```python
from build123d import *

# Parameters (mm, degrees)
SKETCH_R          = 32.25
PAD_DEPTH         = 2.13
SKETCH004_R       = 1.25
SKETCH004_R_2     = 2
POCKET001_DEPTH   = 5
CHAMFER_SIZE      = 1
SKETCH001_R       = 19.2
PAD001_DEPTH      = 1.5
SKETCH003_W       = 13.85
SKETCH003_H       = 6.2
POCKET_DEPTH      = 2.131
POCKET_DEPTH_BACK = 1.501
SKETCH009_R       = 18
POCKET002_DEPTH   = 2
PAD002_DEPTH      = 21


with BuildPart() as part:
    # Sketch → Pad (new body)
    with BuildSketch(Plane.XY):
        Circle(SKETCH_R)
    extrude(amount=PAD_DEPTH)

    # Sketch004 → Pocket001 (cut)
    with BuildSketch(Plane.XY.offset(2.13)):
        with Locations((0, 27)):
            Circle(SKETCH004_R)
        with Locations((19.445436, 19.445436)):
            Circle(SKETCH004_R_2)
        with Locations((27, 0)):
            Circle(SKETCH004_R)
        with Locations((0, -27)):
            Circle(SKETCH004_R)
        with Locations((-19.445436, -19.445436)):
            Circle(SKETCH004_R_2)
        with Locations((-19.445436, 19.445436)):
            Circle(SKETCH004_R_2)
        with Locations((19.445436, -19.445436)):
            Circle(SKETCH004_R_2)
        with Locations((-26.994671, -0.536434)):
            Circle(SKETCH004_R)
    extrude(amount=-POCKET001_DEPTH, mode=Mode.SUBTRACT)

    # Chamfer
    chamfer_edges = [part.edges().sort_by_distance(p)[0] for p in [
        (25.75, 0, 2.13),
        (-1.25, 27, 2.13),
        (-28.244671, -0.536434, 2.13),
        (-1.25, -27, 2.13),
    ]]
    chamfer(chamfer_edges, length=CHAMFER_SIZE)

    # Sketch001 → Pad001 (join)
    with BuildSketch(Plane.XY.offset(2.13)):
        Circle(SKETCH001_R)
    extrude(amount=PAD001_DEPTH)

    # Sketch003 → Pocket (cut, two sides)
    with BuildSketch(Plane.XY.offset(2.13)) as pocket_sk:
        Rectangle(SKETCH003_W, SKETCH003_H)
        with Locations((0, -10.7)):
            Rectangle(SKETCH003_W, SKETCH003_H)
        with Locations((0, 10.7)):
            Rectangle(SKETCH003_W, SKETCH003_H)
    extrude(amount=-POCKET_DEPTH, mode=Mode.SUBTRACT)
    extrude(pocket_sk.sketch, amount=POCKET_DEPTH_BACK, mode=Mode.SUBTRACT)

    # Sketch009 → Pocket002 (cut)
    with BuildSketch(Plane.XY):
        Circle(SKETCH009_R)
    extrude(amount=-POCKET002_DEPTH, mode=Mode.SUBTRACT)

    # Sketch006 → Pad002 (join)
    with BuildSketch(Plane(origin=(0, 0, 0), x_dir=(0.866025, 0.5, 0), z_dir=(0, 0, 1))):
        with BuildLine():
            ThreePointArc((-1.804633, 22.427512), (-19.485572, 11.25), (-20.325112, -9.650898))
            ThreePointArc((-20.325112, -9.650898), (-20.45119, -11.8075), (-18.520479, -12.776614))
            ThreePointArc((-18.520479, -12.776614), (0, -22.5), (18.520479, -12.776614))
            ThreePointArc((18.520479, -12.776614), (20.45119, -11.8075), (20.325112, -9.650898))
            ThreePointArc((20.325112, -9.650898), (19.485572, 11.25), (1.804633, 22.427512))
            ThreePointArc((1.804633, 22.427512), (0, 23.615), (-1.804633, 22.427512))
        make_face()
        with BuildLine():
            ThreePointArc((-1.860528, 21.017812), (-18.273136, 10.55), (-19.132223, -8.897642))
            ThreePointArc((-17.271696, -12.120171), (-17.04771, -9.8425), (-19.132223, -8.897642))
            ThreePointArc((-17.271696, -12.120171), (-16.59064, -13.036896), (-15.860983, -13.915431))
            Line((-14.58548, -11.706194), (-15.860983, -13.915431))
            Line((-13.892659, -12.106194), (-14.58548, -11.706194))
            Line((-15.29504, -14.53519), (-13.892659, -12.106194))
            ThreePointArc((-15.29504, -14.53519), (1.560407, -21.042223), (17.271696, -12.120171))
            ThreePointArc((19.132223, -8.897642), (17.04771, -9.8425), (17.271696, -12.120171))
            ThreePointArc((19.132223, -8.897642), (19.003303, 9.169759), (4.940323, 20.513488))
            Line((4.940323, 20.513488), (3.537942, 18.084493))
            Line((3.537942, 18.084493), (2.845122, 18.484493))
            Line((2.845122, 18.484493), (4.120625, 20.69373))
            ThreePointArc((4.120625, 20.69373), (2.994963, 20.886364), (1.860528, 21.017812))
            ThreePointArc((-1.860528, 21.017812), (0, 19.685), (1.860528, 21.017812))
        make_face(mode=Mode.SUBTRACT)
    extrude(amount=-PAD002_DEPTH)


solid = part.part
```
Can you work these out from the model? Positions are in its coordinate system, mm. A direction names the side the tool comes from. Round coordinates to 2 decimals unless told otherwise and drop trailing zeros. Loops run counter-clockwise (first coordinate to the right, second up) from the corner with the lowest first, then second, coordinate; pieces in that order, holes last. Notation, with made-up numbers: M 82,-36.75 L 107,-36.75 A33 cw 107,-7.75 Z; hole C 8,33 d11. An arc over 180 degrees is marked long. Answer as a JSON object with one key per item and string values. Group by question number.
Q1. Imagine slicing it at A-A, the plane z = -2.75. Please give me the cut outline in (x, y) (3 decimals).
Q2. Will these pins go through, and if not, where does the flat tip stop? pin 1 (8 mm diameter, centred on y = 16, z = -10, fed in from -X); pin 2 (2 mm diameter, centred on y = -19, z = -14, fed in from -X); pin 3 (4.5 mm diameter, centred on x = -19.45, y = -19.45, fed in from +Z).
Q3. On a 3-axis mill with a long thin cutter (end or side, diameter ignored), from which of +Z, -Z, +X, -X, +Y, -Y can I reach the whole of each face in a straight line? I mean faces 3 (the flat face through (-5.978, 19, -10)), 4 (the cylindrical face through (11.513, 19.332, -10.353)), 5 (the flat face through (6.925, -11, 2)), 6 (the cylindrical face through (10.985, -19.636, -10.353)). Say none if no direction works.
Q4. Please list where these lines run through material, in increasing order: L1, parallel to X at y = -19, z = -5.5; L2, parallel to Z at x = 21.5, y = -13; L3, parallel to Z at x = -9, y = 16.
Q5. Imagine slicing it at C-C, the plane y = -27. Please give me the cut outline in (x, z), then the cut area to 3 significant figures.
Q6. We'd pull the mould along X, two halves only. Please class faces 1 (the flat face through (0, -7.6, 2)), 2 (the flat face through (-6.6, -18.8, -21)): +X half, -X half, draft (parallel to the pull), parting line (faces both ways), or undercut.
Q7. Imagine slicing it at B-B, the plane x = -5. Please give me the cut outline in (y, z).
Findings:
{
 "1": {"outline": "M -12.777,-18.52 A1.965 ccw -9.651,-20.325 A22.5 ccw 22.428,-1.805 A1.965 ccw 22.428,1.805 A22.5 ccw -9.651,20.325 A1.965 ccw -12.777,18.52 A22.5 ccw Z; hole M -12.12,-17.272 A1.965 cw -8.898,-19.132 A21.1 ccw -6.778,-19.982 L -6.778,-17.431 L -5.978,-17.431 L -5.978,-20.235 A21.1 ccw 21.018,-1.861 A1.965 cw 21.018,1.861 A21.1 ccw -5.978,20.235 L -5.978,17.431 L -6.778,17.431 L -6.778,19.982 A21.1 ccw -8.898,19.132 A1.965 cw -12.12,17.272 A21.1 ccw Z"},
 "2": {"pin 1": "stops at x = -19.03", "pin 2": "stops at x = -13.5", "pin 3": "stops at z = 2.13"},
 "3": {"face 3": "-Z", "face 4": "-Z, +Y", "face 5": "+Z, -Z", "face 6": "-Z, -Y"},
 "4": {"L1": "x = -12.77 to -8.88, -6.78 to -5.98, 9.18 to 12.05", "L2": "z = 0 to 2.13", "L3": "z = 0 to 3.63"},
 "5": {"outline": "M -17.64,0 L -1.25,0 L -1.25,1.13 L -2.25,2.13 L -17.64,2.13 Z; M 1.25,0 L 17.64,0 L 17.64,2.13 L 2.25,2.13 L 1.25,1.13 Z", "area": "68.8 mm2"},
 "6": {"face 1": "undercut", "face 2": "draft"},
 "7": {"outline": "M -31.86,0 L -21.94,0 L -21.94,-21 L -20.5,-21 L -20.5,0 L -13.8,0 L -13.8,3.63 L -18.54,3.63 L -18.54,2.13 L -31.86,2.13 Z; M -7.6,0 L -3.1,0 L -3.1,3.63 L -7.6,3.63 Z; M 3.1,0 L 7.6,0 L 7.6,3.63 L 3.1,3.63 Z; M 13.8,0 L 20.5,0 L 20.5,-21 L 21.94,-21 L 21.94,0 L 31.86,0 L 31.86,2.13 L 18.54,2.13 L 18.54,3.63 L 13.8,3.63 Z"}
}
